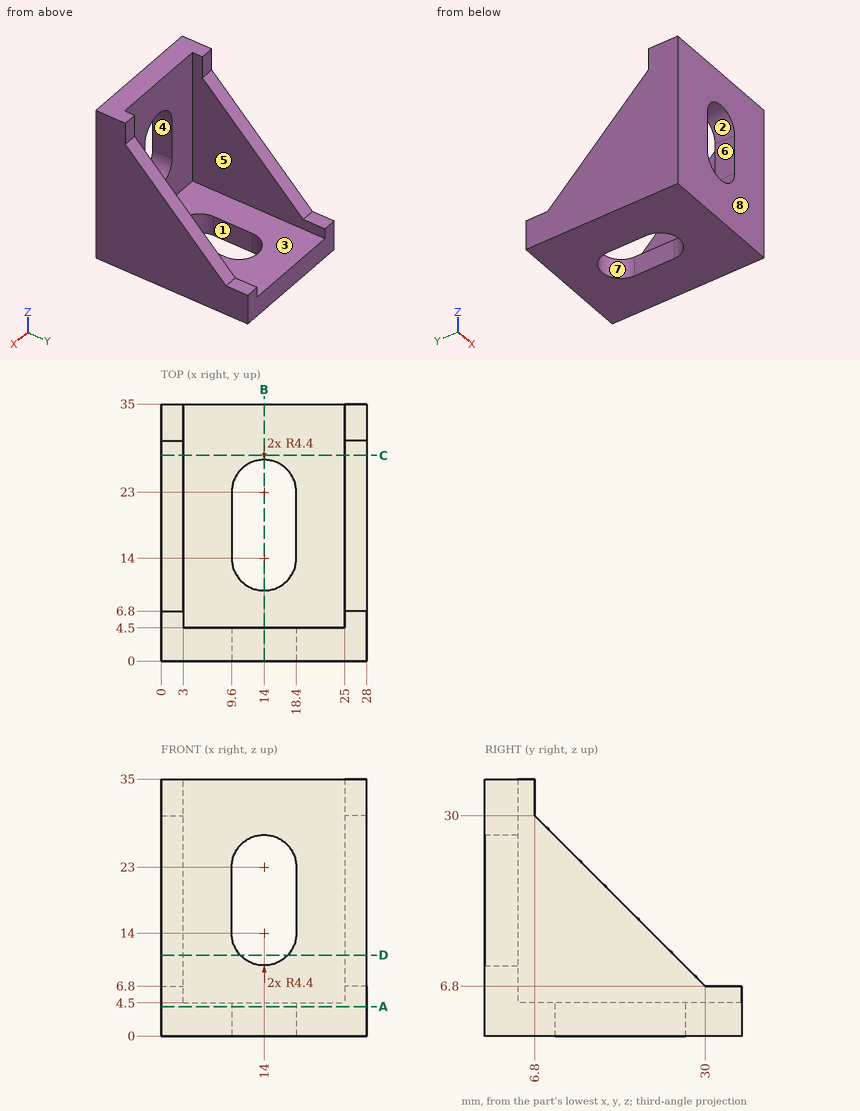
Study the drawing (mm; zero at the part's minimum x, y, z) and answer. A direction names the side the tool comes from. Round coordinates to 2 decimals unless told otherwise and drop trailing zeros. Loops run counter-clockwise (first coordinate to the right, second up) from the corner with the lowest first, then second, coordinate; pieces in that order, holes last.
Q1. Section B-B, the plane x = 14 is taken. Determine the outline of the cut face in (y, z), then the cut area to 3 significant figures.
Q2. Section A-A, the plane z = 4 is taken. Determine the outline of the cut face in (x, y).
Q3. Given pin 1 Ø2.5 at (x, y) = (26, 32) entering from +Z; pin 2 Ø6.5 at (x, y) = (9.5, 19) entering from +Z; pin 3 Ø10 at (x, z) = (24, 17) entering from +Y, each flat-ended and moving along its own axis, determine where each tip first touches the part or whether it passes through.
Q4. Find the intervals of material crossed by line 1 (X direction, y = 20, z = 5); line 2 (X direction, y = 3, z = 19.5); line 3 (Z direction, x = 12.25, y = 8.5), in increasing order.
Q5. For a pull along Z with two mould halves and no side action, classify the marked faces 1, 2, 3 and 4 as released by +Z, released by -Z, zero draft, split by the parting line, or undercut.
Q6. Which of the six approach directions +Z, -Z, +X, -X, +Y, -Y give full straight-line access (tool end or side, diameter ignored) to the marked faces 5, 6, 7 and 8?
Q7. Section D-D, the plane z = 11 is taken. Determine the outline of the cut face in (x, y), then the cut area to 3 significant figures.
Q8. Section C-C, the plane y = 28 is taken. Determine the outline of the cut face in (x, z).
Completed:
1. outline: (0, 0) - (9.6, 0) - (9.6, 4.5) - (4.5, 4.5) - (4.5, 9.6) - (0, 9.6) - close; (0, 27.4) - (4.5, 27.4) - (4.5, 35) - (0, 35) - close; (27.4, 0) - (35, 0) - (35, 4.5) - (27.4, 4.5) - close
1. area: 135 mm2
2. outline: (0, 0) - (28, 0) - (28, 35) - (0, 35) - close; hole (9.6, 14) arc R4.4 ccw to (18.4, 14) - (18.4, 23) arc R4.4 ccw to (9.6, 23) - close
3. pin 1: stops at z = 6.8
3. pin 2: stops at z = 4.5
3. pin 3: stops at y = 24.7
4. line 1: x = 0 to 3, 25 to 28
4. line 2: x = 0 to 9.6, 18.4 to 28
4. line 3: z = 0 to 4.5
5. face 1: zero draft
5. face 2: undercut
5. face 3: released by +Z
5. face 4: undercut
6. face 5: +Z, +Y
6. face 6: +Y, -Y
6. face 7: +Z, -Z
6. face 8: +Z, -Z, +X, -X, -Y
7. outline: (0, 0) - (10.78, 0) - (10.78, 4.5) - (3, 4.5) - (3, 25.8) - (0, 25.8) - close; (17.22, 0) - (28, 0) - (28, 25.8) - (25, 25.8) - (25, 4.5) - (17.22, 4.5) - close
7. area: 225 mm2
8. outline: (0, 0) - (28, 0) - (28, 8.8) - (25, 8.8) - (25, 4.5) - (3, 4.5) - (3, 8.8) - (0, 8.8) - close
